Verification items for the finished model (mm, model axes). A direction names the side the tool comes from. Round coordinates to 2 decimals unless told otherwise and drop trailing zeros. Write each loop counter-clockwise with the first axis right and the second up, starting at its lowest first coordinate (ties: lowest second). Pieces come first, ordered by that corner, then holes. Notation, with made-up numbers: M -3,56.5 L 22,56.5 A9 ccw 22,69.5 Z; hole C -10.5,68 d7. An arc over 180 degrees is marked long. One line per question, with ' | ' between items. Start each with the question number.
Q1. Cross-section at A-A (x = -51). Record the boundary of the cut face in (y, z).
Q2. Thickness scan on line 1 along X through (y, z) = (10.25, -4); line 2 along Z through (x, y) = (-24, 5.75); line 3 along X through (y, z) = (7, -4). Record the ranges inside material, lowest first. Write a range as from..to.
Q3. Tool access check on faces 1 (the face through (-51, 8, -20)), 2 (the face through (-94.48, 7.67, -8.57)). Record the directions out of +Z, -Z, +X, -X, +Y, -Y that give a thin tool (end or side, any length) a straight path to the whole face; none if there is none.
Q4. Release check for a two-part mould opening along X. For faces 3 (the face through (-3, 8, -18)), 4 (the face through (-8, 8, 0)), 5 (the face through (-93.55, 7.8, -1.43)) record: released by +X, released by -X, zero draft, split by the parting line, or undercut.
Q5. Gauge pin test, flat end, axial feed: pin 1 (5 mm diameter, centred on x = -48.5, y = 10.5, fed in from +Z). Record the tip position at first contact, or that the pin passes through.
Q6. Cross-section at B-B (z = -7.5). Record the boundary of the cut face in (x, y), then the cut area to 3 significant figures.
from build123d import *

# Parameters (mm, degrees)
SKETCH2_R             = 2.5
BOSS_EXTRUDE1_DEPTH   = 15
BOSS_EXTRUDE1_2_DEPTH = 15
SKETCH3_W             = 94
SKETCH3_H             = 10
BOSS_EXTRUDE2_DEPTH   = 5
FILLET1_R             = 2
FILLET2_R             = 0.4
CHAMFER1_SIZE         = 4
CHAMFER1_SIZE2        = 1.455880937
CHAMFER1_PART_2_SIZE  = 4
CHAMFER1_PART_2_SIZE2 = 1.455880937
FILLET4_R             = 1.5


with BuildPart() as part:
    # Sketch2 → Boss-Extrude1 (new body)
    with BuildSketch(Plane(origin=(0, 0, 0), x_dir=(0, 1, 0), z_dir=(0, 0, 1))):
        with Locations((8, 92)):
            Circle(SKETCH2_R)
    extrude(amount=-BOSS_EXTRUDE1_DEPTH)



with BuildPart() as body_2:
    # Sketch2 → Boss-Extrude1 2 (new body)
    with BuildSketch(Plane(origin=(0, 0, 0), x_dir=(0, 1, 0), z_dir=(0, 0, 1))):
        with Locations((8, 8)):
            Circle(SKETCH2_R)
    extrude(amount=-BOSS_EXTRUDE1_2_DEPTH)


with BuildPart() as part_1:
    add(part.part)

    add(body_2.part)  # Boss-Extrude2 merges body 2
    # Sketch3 → Boss-Extrude2 (add)
    with BuildSketch(Plane(origin=(0, 0, -15), x_dir=(1, 0, 0), z_dir=(0, 0, -1))):
        with Locations((-50, -8)):
            Rectangle(SKETCH3_W, SKETCH3_H)
    extrude(amount=BOSS_EXTRUDE2_DEPTH)

    # Fillet1
    fillet1_edges = [part_1.edges().sort_by_distance(p)[0] for p in [
        (-8, 5.5, -15),
        (-92, 5.5, -15),
    ]]
    fillet(fillet1_edges, radius=FILLET1_R)

    # Fillet2
    fillet2_edges = [part_1.edges().sort_by_distance(p)[0] for p in [
        (-97, 8, -15),
        (-50, 13, -15),
        (-3, 8, -15),
        (-50, 3, -15),
    ]]
    fillet(fillet2_edges, radius=FILLET2_R)

    # Chamfer1
    chamfer1_edges = [part_1.edges().sort_by_distance(p)[0] for p in [
        (-8, 5.5, 0),
    ]]
    chamfer1_side = [part_1.faces().sort_by_distance(p)[0] for p in [
        (-8, 5.5, -6.5),
    ]]
    chamfer(chamfer1_edges, length=CHAMFER1_SIZE, length2=CHAMFER1_SIZE2, reference=chamfer1_side[0])

    # Chamfer1 part 2
    chamfer1_part_2_edges = [part_1.edges().sort_by_distance(p)[0] for p in [
        (-92, 5.5, 0),
    ]]
    chamfer1_part_2_side = [part_1.faces().sort_by_distance(p)[0] for p in [
        (-92, 5.5, -6.5),
    ]]
    chamfer(chamfer1_part_2_edges, length=CHAMFER1_PART_2_SIZE, length2=CHAMFER1_PART_2_SIZE2, reference=chamfer1_part_2_side[0])

    # Fillet4
    fillet4_edges = [part_1.edges().sort_by_distance(p)[0] for p in [
        (-8, 5.5, -4),
        (-92, 5.5, -4),
    ]]
    fillet(fillet4_edges, radius=FILLET4_R)


solid = part_1.part
Determined:
1) outline: M 3,-20 L 13,-20 L 13,-15.4 A0.4 ccw 12.6,-15 L 3.4,-15 A0.4 ccw 3,-15.4 Z
2) line 1: x = -93.03..-90.97, -9.03..-6.97 | line 2: z = -20..-15 | line 3: x = -94.27..-89.73, -10.27..-5.73
3) face 1: -Z, +X, -X, +Y, -Y | face 2: +Z
4) face 3: released by +X | face 4: zero draft | face 5: undercut
5) pin 1: stops at z = -15
6) outline: C -92,8 d5; C -8,8 d5 | area: 39.3 mm²
